from build123d import *

# Parameters (mm, degrees)
SKETCH1_R           = 10
BOSS_EXTRUDE1_DEPTH = 10
SKETCH3_R           = 4
BOSS_EXTRUDE2_DEPTH = 7
SKETCH4_R           = 2.2
CUT_EXTRUDE1_DEPTH  = 18


with BuildPart() as part:
    # Sketch1 → Boss-Extrude1 (new body)
    with BuildSketch(Plane.XY):
        Circle(SKETCH1_R)
    extrude(amount=BOSS_EXTRUDE1_DEPTH)

    # Sketch2 → Cut-Revolve2 (revolve, cut)
    with BuildSketch(Plane(origin=(0, 0, 0), x_dir=(0, 0, -1), z_dir=(1, 0, 0))):
        Polygon((0, -10), (-10, -4), (-10, -10), align=None)
    revolve(axis=Axis((0, 0, 10), (0, 0, -1)), mode=Mode.SUBTRACT)

    # Sketch3 → Boss-Extrude2 (add)
    with BuildSketch(Plane.XY.offset(10)):
        Circle(SKETCH3_R)
    extrude(amount=BOSS_EXTRUDE2_DEPTH)

    # Sketch4 → Cut-Extrude1 (cut, through all)
    with BuildSketch(Plane.XY.offset(17)):
        Circle(SKETCH4_R)
    extrude(amount=-CUT_EXTRUDE1_DEPTH, mode=Mode.SUBTRACT)


solid = part.part
Can you work these out from the model? Positions are in its coordinate system, mm. A direction names the side the tool comes from. Give positions to 0.01 mm unless a question says otherwise; leave off trailing zeros. Loops run counter-clockwise (first coordinate to the right, second up) from the corner with the lowest first, then second, coordinate; pieces in that order, holes last. Notation, with made-up numbers: (37.25, 84.25) - (62.25, 84.25) arc R23 ccw to (62.25, 110.25) - close; hole circle Ø4 at (-26.75, -27). An arc over 180 degrees is marked (long way). Return JSON: item names as keys, results as strings.
1. We'd pull the mould along X, two halves only. Please class faces 3 (the face through (-1.49, -4.73, 8.4)), 4 (the face through (2.1, 0.66, 8.62)), 5 (the face through (2, -2, 17)): +X half, -X half, draft (parallel to the pull), parting line (faces both ways), or undercut.
Output values:
{"face 3": "parting line", "face 4": "undercut", "face 5": "draft"}
2. I want a section at C-C on z = 7.25. Please give me the cut outline in (x, y).
Output values:
{"outline": "circle Ø11.3 at (0, 0); hole circle Ø4.4 at (0, 0)"}
3. If I drill on line 1 (Y direction, x = 0, z = 10.75); line 2 (X direction, y = -1.25, z = 10.75), over which ranges is the centre line in solid material (lowest first)?
Output values:
{"line 1": "y = -4 to -2.2, 2.2 to 4", "line 2": "x = -3.8 to -1.81, 1.81 to 3.8"}
4. I want a section at A-A on x = 0. Please give me the cut outline in (y, z), and give its area (3 significant figures).
Output values:
{"outline": "(-10, 0) - (-2.2, 0) - (-2.2, 17) - (-4, 17) - (-4, 10) - close; (2.2, 0) - (10, 0) - (4, 10) - (4, 17) - (2.2, 17) - close", "area": "121 mm²"}
5. I want a section at D-D on z = 15.25. Please give me the cut outline in (x, y), and give its area (3 significant figures).
Output values:
{"outline": "circle Ø8 at (0, 0); hole circle Ø4.4 at (0, 0)", "area": "35.1 mm²"}
6. For faces 1 (the face through (-0.867, -3.905, 13.451)), 2 (the face through (-0.1, 2.4, 0)), which set-ups out of +Z, -Z, +X, -X, +Y, -Y let a thin tool reach every point of the face, with its end or its side?
Output values:
{"face 1": "+Z", "face 2": "-Z, +X, -X, +Y, -Y"}
7. I'm going to push flat-ended pins straight in: pin 1 Ø3 at (x, z) = (0.5, 11.5) entering from -Y; pin 2 Ø8 at (y, z) = (1, 8.5) entering from -X; pin 3 Ø3 at (x, z) = (0.5, 11) entering from -Y. Where does each tip first touch, or does it pass through?
Output values:
{"pin 1": "stops at y = -4", "pin 2": "stops at x = -7.26", "pin 3": "stops at y = -4.28"}
